from build123d import *

# Parameters (mm, degrees)
SKETCH1_R                = 100
BOSS_EXTRUDE1_DEPTH      = 3.175
FILLET1_R                = 3
CIRPATTERN1_COUNT        = 2
FILLET1_OF_CIRPATTERN1_R = 3
SKETCH2_R                = 2.65
CUT_EXTRUDE1_DEPTH       = 174.229104079
CIRPATTERN2_COUNT        = 8
LIGHTENING_CUT_DEPTH     = 174.229104079
LIGHTENING_PATTERN_COUNT = 8


with BuildPart() as part:
    # Sketch1 → Boss-Extrude1 (new, symmetric)
    with BuildSketch(Plane(origin=(0, 0, 0), x_dir=(1, 0, 0), z_dir=(0, 1, 0))):
        with BuildLine():
            Line((-111.986312116, 1.750970805), (-132, 0))
            ThreePointArc((-132, 0), (-115.815804966, -46.398149165), (-79.477414809, -79.477414809))
            ThreePointArc((-79.477414809, -79.477414809), (-78.32708198, -80.19539315), (-77.284459499, -81.062397694))
            ThreePointArc((-77.284459499, -81.062397694), (103.297481806, 43.285450818), (-111.986312116, 1.750970805))
        make_face()
        with Locations(Location((0, 0, 0), (0, 0, 270))):
            Circle(SKETCH1_R, mode=Mode.SUBTRACT)
    boss_extrude1 = extrude(amount=BOSS_EXTRUDE1_DEPTH, both=True)

    # Fillet1
    fillet1_edges = [part.edges().sort_by_distance(p)[0] for p in [
        (-111.986312116, 0, -1.750970805),
    ]]
    fillet(fillet1_edges, radius=FILLET1_R)

    # CirPattern1: Boss-Extrude1 ×2 about axis
    cirpattern1_axis = Axis((0, 0, 0), (0, 1, 0))
    for i in range(1, CIRPATTERN1_COUNT):
        add(boss_extrude1.rotate(cirpattern1_axis, i * 360 / CIRPATTERN1_COUNT))

    # Fillet1 of CirPattern1
    fillet1_of_cirpattern1_edges = [part.edges().sort_by_distance(p)[0] for p in [
        (111.986312116, 0, 1.750970805),
    ]]
    fillet(fillet1_of_cirpattern1_edges, radius=FILLET1_OF_CIRPATTERN1_R)

    # Sketch2 → Cut-Extrude1 (cut, through all)
    with BuildSketch(Plane(origin=(0, 3.175, 0), x_dir=(1, 0, 0), z_dir=(0, 1, 0))):
        with Locations(Location((-102.388137587, -27.434818781, 0), (0, 0, 270))):
            Circle(SKETCH2_R)
    cut_extrude1 = extrude(amount=-CUT_EXTRUDE1_DEPTH, mode=Mode.SUBTRACT)

    # CirPattern2: Cut-Extrude1 ×8 about axis
    cirpattern2_axis = Axis((0, 0, 0), (0, 1, 0))
    for i in range(1, CIRPATTERN2_COUNT):
        add(cut_extrude1.rotate(cirpattern2_axis, i * 360 / CIRPATTERN2_COUNT), mode=Mode.SUBTRACT)

    # Sketch3 → Lightening Cut (cut, through all)
    with BuildSketch(Plane(origin=(0, 3.175, 0), x_dir=(1, 0, 0), z_dir=(0, 1, 0))):
        with BuildLine():
            ThreePointArc((-101.318921825, 37.396204088), (-107.076045028, 14.09682876), (-107.545413115, -9.898692736))
            ThreePointArc((-107.545413115, -9.898692736), (-105.370522266, -11.706965335), (-103.562249667, -9.532074486))
            ThreePointArc((-103.562249667, -9.532074486), (-103.110265583, 13.574723991), (-97.566369165, 36.011159492))
            ThreePointArc((-97.566369165, 36.011159492), (-98.750123197, 38.57995812), (-101.318921825, 37.396204088))
        make_face()
    lightening_cut = extrude(amount=-LIGHTENING_CUT_DEPTH, mode=Mode.SUBTRACT)

    # Lightening Pattern: Lightening Cut ×8 about axis
    lightening_pattern_axis = Axis((0, 0, 0), (0, 1, 0))
    for i in range(1, LIGHTENING_PATTERN_COUNT):
        add(lightening_cut.rotate(lightening_pattern_axis, i * 360 / LIGHTENING_PATTERN_COUNT), mode=Mode.SUBTRACT)


solid = part.part
Model file for the job. Use its own axes, mm. A direction names the side the tool comes from. Give positions to 0.01 mm unless a question says otherwise; leave off trailing zeros. Answer as CSV lines item,"result".
1. Drill centre lines: L1, parallel to X at y = 2, z = -77; L2, parallel to X at y = 1, z = 65.5; L3, parallel to Z at x = 24, y = -1.5. Where is each one in solid material? Low to high. Write a range as [from, to].
Responses:
L1,"x = [-81.33, -75.73], [-69.91, -63.8], [63.8, 69.91], [75.73, 83.85]"
L2,"x = [-99.39, -85.87], [-80.78, -75.56], [75.56, 90.85]"
L3,"z = [-109.4, -105.3], [-101.19, -97.08], [97.08, 109.4]"
2. 3-axis set-ups, long thin cutter, end or side, ignore diameter. For faces 1 (the face through (-40.394, 0.044, -104.462)), 2 (the face through (-13.253, 0.044, 103.152)): which of +Z, -Z, +X, -X, +Y, -Y reach the whole face in a straight line?
Responses:
face 1,"-Z, +Y, -Y"
face 2,"+Y, -Y"
3. Band-saw the part on A-A (y = 0). Count the separate pieces of the cut face and the enclosed holes in it, and give its area (3 significant figures).
Responses:
separate pieces,"1"
enclosed holes,"17"
area,"8,440 mm2"
4. Pin check, flat tips, straight feed: pin 1 (4 mm diameter, centred on x = 95, z = 27, fed in from -Y) (3 decimals); pin 2 (2 mm diameter, centred on x = -51, y = 1.5, fed in from +Z); pin 3 (2 mm diameter, centred on y = -1, z = 32, fed in from +X). Stop position of each tip, or through.
Responses:
pin 1,"stops at y = -3.175"
pin 2,"stops at z = 100.22"
pin 3,"stops at x = 107.62"
5. Two-plate mould, pull along X, no slides. Class faces 3 (the face through (-65.479, 0.044, -85.887)), 4 (the face through (40, 3.175, 92)), 5 (the face through (116.197, 0.044, -45.817)): +X half, -X half, draft (parallel to the pull), parting line (faces both ways), or undercut.
Responses:
face 3,"undercut"
face 4,"draft"
face 5,"+X half"
